Geometry: final body of the model. Coordinates: model frame, mm. Give positions to 0.01 mm unless a question says otherwise; leave off trailing zeros. Write each loop counter-clockwise with the first axis right and the second up, starting at its lowest first coordinate (ties: lowest second). Pieces come first, ordered by that corner, then holes. Notation, with made-up numbers: M 45,72.25 L 88,72.25 A24 ccw 88,99.25 Z; hole C -26,45 d9. An arc over 180 degrees is marked long. Use a Markdown table: item, result. Add a question column.
1) Section A-A on z = 0. Return the cut outline in (x, y) (3 decimals), then the cut area to 3 significant figures.
2) Section C-C on y = -0.6. State how many separate pieces and enclosed holes the cut face has, then the cut area to 3 significant figures.
3) Pin query (flat end, axial travel): pin 1 (13.5 mm diameter, centred on x = 117.33, z = -48.6, fed in from +Y); pin 2 (1.5 mm diameter, centred on x = -76, y = -3, fed in from -Z); pin 3 (1 mm diameter, centred on y = -2.5, z = 76.5, fed in from +X); pin 4 (2 mm diameter, centred on y = -2, z = -63.5, fed in from +X). Return the tip coordinate at first contact, or that it passes through.
4) Section B-B on x = 0. Return the cut outline in (y, z) (3 decimals), then the cut area to 3 significant figures.
5) Line query: line 1 (X direction, y = -2.15, z = 88); line 2 (Z direction, x = -124, y = -1.95); line 3 (X direction, y = -0.6, z = 31.5). Output: solid intervals per line, ascending.
```python
from build123d import *

# Parameters (mm, degrees)
SKETCH1_R               = 142.875
SKETCH1_R_2             = 11.25
BOSS_EXTRUDE2_DEPTH     = 3.81
SKETCH2_R               = 11.25
CUT_EXTRUDE1_DEPTH      = 203.091680556
CUT_EXTRUDE2_DEPTH      = 203.091680556
CUT_EXTRUDE2_DEPTH_BACK = 203.091680556
SKETCH4_R               = 111.125
CIRPATTERN1_COUNT       = 32


with BuildPart() as part:
    # Sketch1 → Boss-Extrude2 (new body)
    with BuildSketch(Plane(origin=(0, 0, 0), x_dir=(1, 0, 0), z_dir=(0, 1, 0))):
        with Locations(Location((0, 0, 0), (0, 0, 270))):
            Circle(SKETCH1_R)
        with Locations(Location((0, 0, 0), (0, 0, 270))):
            Circle(SKETCH1_R_2, mode=Mode.SUBTRACT)
    extrude(amount=-BOSS_EXTRUDE2_DEPTH)

    # Sketch2 → Cut-Extrude1 (cut, through all)
    with BuildSketch(Plane(origin=(0, 0, 0), x_dir=(1, 0, 0), z_dir=(0, 1, 0))):
        with Locations(Location((-127, 0, 0), (0, 0, 270))):
            Circle(SKETCH2_R)
    cut_extrude1 = extrude(amount=-CUT_EXTRUDE1_DEPTH, mode=Mode.SUBTRACT)

    # Sketch4 → Cut-Extrude2 (cut, two sides: drawn at the far end of the back side and taken through both)
    with BuildSketch(Plane(origin=(0, 0, 0), x_dir=(1, 0, 0), z_dir=(0, 1, 0)).offset(-CUT_EXTRUDE2_DEPTH_BACK)):
        with Locations(Location((0, 0, 0), (0, 0, 270))):
            Circle(SKETCH4_R)
    extrude(amount=CUT_EXTRUDE2_DEPTH + CUT_EXTRUDE2_DEPTH_BACK, mode=Mode.SUBTRACT)

    # CirPattern1: Cut-Extrude1 ×32 about axis
    cirpattern1_axis = Axis((0, 0, 0), (0, 1, 0))
    for i in range(1, CIRPATTERN1_COUNT):
        add(cut_extrude1.rotate(cirpattern1_axis, i * 360 / CIRPATTERN1_COUNT), mode=Mode.SUBTRACT)


solid = part.part
```
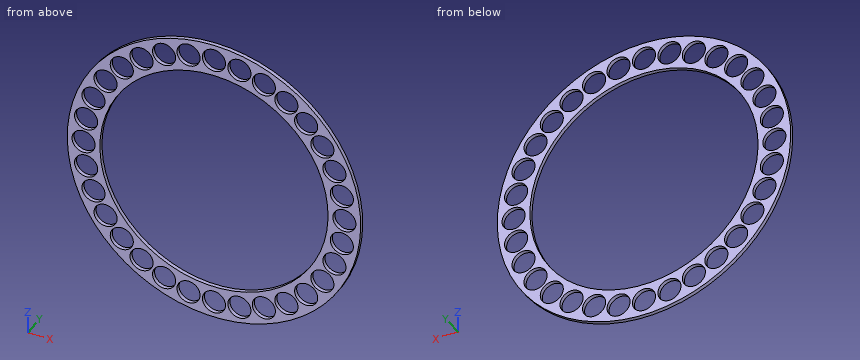
Found:
| question | item | result |
|---|---|---|
| 1 | outline | M -142.875,-3.81 L -138.25,-3.81 L -138.25,0 L -142.875,0 Z; M -115.75,-3.81 L -111.125,-3.81 L -111.125,0 L -115.75,0 Z; M 111.125,-3.81 L 115.75,-3.81 L 115.75,0 L 111.125,0 Z; M 138.25,-3.81 L 142.875,-3.81 L 142.875,0 L 138.25,0 Z |
| 1 | area | 70.5 mm² |
| 2 | separate pieces | 1 |
| 2 | enclosed holes | 33 |
| 2 | area | 12,600 mm² |
| 3 | pin 1 | through |
| 3 | pin 2 | z = -121.45 |
| 3 | pin 3 | x = 120.98 |
| 3 | pin 4 | x = 128.48 |
| 4 | outline | M -3.81,-142.875 L 0,-142.875 L 0,-138.25 L -3.81,-138.25 Z; M -3.81,-115.75 L 0,-115.75 L 0,-111.125 L -3.81,-111.125 Z; M -3.81,111.125 L 0,111.125 L 0,115.75 L -3.81,115.75 Z; M -3.81,138.25 L 0,138.25 L 0,142.875 L -3.81,142.875 Z |
| 4 | area | 70.5 mm² |
| 5 | line 1 | -112.56 to -100.91, -78.7 to -67.86, 67.86 to 78.7, 100.91 to 112.56 |
| 5 | line 2 | -70.97 to -57.66, -39.54 to -36.01, -13.54 to -10.84, 10.84 to 13.54, 36.01 to 39.54, 57.66 to 70.97 |
| 5 | line 3 | -139.36 to -133.58, -115.54 to -106.57, 106.57 to 115.54, 133.58 to 139.36 |
